Check sheet for the modelled part. Datum: model origin and axes. Units: mm. Face numbers are marked on the shaded views. Coordinates: 2 decimals unless noted, no trailing zeros. Write each loop counter-clockwise with the first axis right and the second up, starting at its lowest first coordinate (ties: lowest second). Pieces come first, ordered by that corner, then holes. Notation, with made-up numbers: (4, 56.5) - (28, 56.5) arc R12 ccw to (28, 69.5) - close; hole circle Ø4 at (-32.75, -17.75). An arc over 180 degrees is marked (long way). Answer as CSV lines item,"result". Start each with the question number.
from build123d import *

# Parameters (mm, degrees)
SKETCH1_W           = 200
SKETCH1_H           = 240
BASE_DEPTH          = 50
SKETCH2_R           = 26
LOAD_CELL_CUT_DEPTH = 18.6
WIRE_CUT_REACH      = 202
SKETCH3_W           = 35
SKETCH3_H           = 18
WIRE_CUT_FILLET_R   = 5


with BuildPart() as part:
    # Sketch1 → base (new body)
    with BuildSketch(Plane(origin=(0, 0, 0), x_dir=(1, 0, 0), z_dir=(0, 1, 0))):
        Rectangle(SKETCH1_W, SKETCH1_H)
    extrude(amount=BASE_DEPTH)

    # Sketch2 → load cell cut (cut)
    with BuildSketch(Plane(origin=(0, 50, 0), x_dir=(1, 0, 0), z_dir=(0, 1, 0))):
        Circle(SKETCH2_R)
    extrude(amount=-LOAD_CELL_CUT_DEPTH, mode=Mode.SUBTRACT)

    # Sketch3 → wire cut (cut, up to next)
    with BuildSketch(Plane(origin=(-100, 0, 0), x_dir=(0, 0, -1), z_dir=(1, 0, 0)), mode=Mode.PRIVATE) as wire_cut_sk1:
        with Locations((0, 41)):
            Rectangle(SKETCH3_W, SKETCH3_H)
    wire_cut_tool1 = extrude(wire_cut_sk1.sketch, amount=WIRE_CUT_REACH, mode=Mode.PRIVATE) & part.part
    add(wire_cut_tool1.solids().sort_by_distance((-100, 41, 0))[0], mode=Mode.SUBTRACT)

    # wire cut fillet
    wire_cut_fillet_edges = [part.edges().sort_by_distance(p)[0] for p in [
        (-59.614442262, 32, -17.5),
        (-59.614442262, 32, 17.5),
    ]]
    fillet(wire_cut_fillet_edges, radius=WIRE_CUT_FILLET_R)


solid = part.part
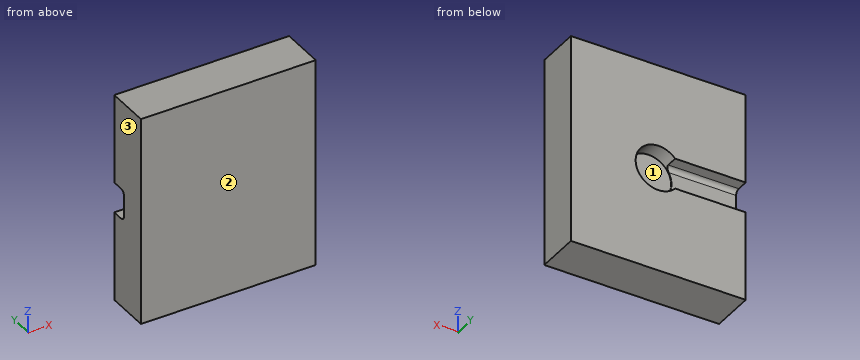
(1) Material ranges on probe 1 along Z at (x, y) = (-27, 38.5); probe 2 along Z at (x, y) = (0, 45); probe 3 along Y at (x, z) = (-20.5, -6), recorded low to high. Write a range as from..to.
(2) Cross-section at C-C on x = 0. Record the boundary of the cut face in (y, z), plus the area to 3 significant figures.
(3) Release check for a two-part mould opening along X. For the marked faces 1, 2 and 3 record: pulls with the +X half, pulls with the -X half, needs draft (parallel to the pull), parting line crosses it, or undercut.
(4) Cross-section at B-B on z = 0. Record the boundary of the cut face in (x, y), plus the area to 3 significant figures.
(5) Cross-section at A-A on x = -66. Record the boundary of the cut face in (y, z).
(6) Go/stop test with a flat-tipped pin: P1, Ø7.5, axis at x = -73, z = -6, coming from the +Y side. Record where the tip stops, or that it passes through.
Checked values:
1,probe 1,"-120..-17.5, 17.5..120"
1,probe 2,"-120..-26, 26..120"
1,probe 3,"0..31.4"
2,outline,"(0, -120) - (50, -120) - (50, -26) - (31.4, -26) - (31.4, 26) - (50, 26) - (50, 120) - (0, 120) - close"
2,area,"11,000 mm^2"
3,face 1,"undercut"
3,face 2,"needs draft"
3,face 3,"pulls with the -X half"
4,outline,"(-100, 0) - (100, 0) - (100, 50) - (26, 50) - (26, 31.4) - (-26, 31.4) - (-26, 32) - (-100, 32) - close"
4,area,"7,700 mm^2"
5,outline,"(0, -120) - (50, -120) - (50, -17.5) - (37, -17.5) arc R5 cw to (32, -12.5) - (32, 12.5) arc R5 cw to (37, 17.5) - (50, 17.5) - (50, 120) - (0, 120) - close"
6,P1,"y = 32"
